Input: part model. Units: mm. Frame: model coordinates. A direction names the side the tool comes from. Round coordinates to 2 decimals unless told otherwise and drop trailing zeros. Order: outer loops, then holes, each group sorted by start corner. A loop starts at its lowest first (then second) coordinate and runs counter-clockwise, first axis right, second up. Notation, with made-up numbers: (-17, 64.5) -> (37, 64.5) arc R15 ccw to (37, 78.5) -> close; hole circle Ø8 at (48.25, 65.25). An arc over 180 degrees is marked (long way). Answer as CSV lines item,"result". Start each with the question number.
1) First-contact query: P1, Ø2, axis at x = 28, y = 14.5, coming from the -Z side; P2, Ø1.5, axis at x = 7, z = -3.5, coming from the -Y side; P3, Ø1.5, axis at x = -23.5, z = -2, coming from the +Y side. Flat tips, straight axial feed; report the tip coordinate or a pass-through.
2) Line query: L1, parallel to Z at x = -25.5, y = -20; L2, parallel to X at y = -14.5, z = -0.75; L3, parallel to Y at x = -9, z = 3. Output: solid intervals per line, ascending.
3) Section query D-D, the plane z = -5.5. Output: boundary loops of the cut face in (x, y).
4) Access query for faces 1 (the face through (5, 30, 0)), 2 (the face through (0, 0, 6.35)). Directions: +Z, -Z, +X, -X, +Y, -Y. A direction counts if a zero-diameter tool reaches every point of the face in a straight line with its end or side. Return the directions, or none.
5) Section query C-C, the plane z = 1.5. Output: boundary loops of the cut face in (x, y) (1 decimal), and give its area (3 significant figures).
```python
from build123d import *

# Parameters (mm, degrees)
SKETCH1_R           = 30.0863
BOSS_EXTRUDE1_DEPTH = 6.35
SKETCH2_R           = 36.5125
BOSS_EXTRUDE2_DEPTH = 6.35
CHAMFER1_SIZE       = 3.175
CHAMFER2_SIZE       = 2.54


with BuildPart() as part:
    # Sketch1 → Boss-Extrude1 (new body)
    with BuildSketch(Plane.XY):
        Circle(SKETCH1_R)
    extrude(amount=-BOSS_EXTRUDE1_DEPTH)

    # Sketch2 → Boss-Extrude2 (add)
    with BuildSketch(Plane.XY):
        Circle(SKETCH2_R)
    extrude(amount=BOSS_EXTRUDE2_DEPTH)

    # Chamfer1
    chamfer1_edges = [part.edges().sort_by_distance(p)[0] for p in [
        (-36.5125, 0, 6.35),
    ]]
    chamfer(chamfer1_edges, length=CHAMFER1_SIZE)

    # Chamfer2
    chamfer2_edges = [part.edges().sort_by_distance(p)[0] for p in [
        (-30.0863, 0, -6.35),
    ]]
    chamfer(chamfer2_edges, length=CHAMFER2_SIZE)


solid = part.part
```
Findings:
1,P1,"stops at z = 0"
1,P2,"stops at y = -29.43"
1,P3,"stops at y = 19.69"
2,L1,"z = 0 to 6.35"
2,L2,"x = -26.36 to 26.36"
2,L3,"y = -35.39 to 35.39"
3,outline,"circle Ø56.79 at (0, 0)"
4,face 1,"-Z"
4,face 2,"+Z, +X, -X, +Y, -Y"
5,outline,"circle Ø73 at (0, 0)"
5,area,"4,190 mm^2"
